Can you work these out from the drawing? Everything is in mm from the part's minimum corner. A direction names the side the tool comes from. Round coordinates to 2 decimals unless told otherwise and drop trailing zeros. Order: outer loops, then holes, each group sorted by start corner. A loop starts at its lowest first (then second) coordinate and runs counter-clockwise, first axis right, second up. Notation, with made-up numbers: M -24,65 L 5,65 A22 ccw 5,72 Z; hole C 26.25,-19 d11. An arc over 180 degrees is marked long. Write each question's results on one line, items separated by ' | '. Start each with the question number.
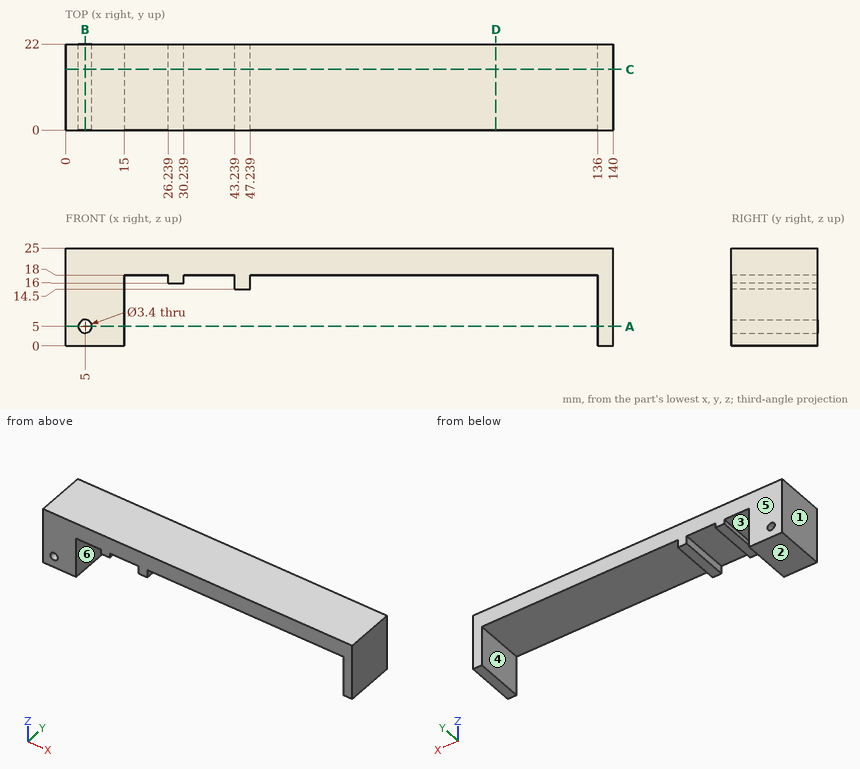
(1) I'm going to push flat-ended pins straight in: pin 1 Ø10.5 at (x, y) = (38.5, 14.5) entering from -Z; pin 2 Ø12.5 at (x, y) = (22, 14.5) entering from -Z; pin 3 Ø11 at (x, y) = (105.5, 7) entering from -Z. Where does each tip first touch, or does it pass through?
(2) I want a section at C-C on y = 15.5. Write out the boundary of the cut face in (x, z), and give its area (3 significant figures).
(3) If we mould it in two halves opening along X, with no side actions, what happens to the marked faces 1, 2, 3 and 4? For each: pulls with the +X half, pulls with the -X half, needs draft (parallel to the pull), parting line crosses it, or undercut.
(4) Please list where these lines run through material, in increasing order: line 1 (X direction, y = 16, z = 14.75); line 2 (Z direction, x = 5, y = 13.5); line 3 (X direction, y = 17.5, z = 7.25).
(5) I want a section at D-D on x = 110. Write out the boundary of the cut face in (y, z).
(6) I want a section at A-A on z = 5. Write out the boundary of the cut face in (x, y), and give its area (3 significant figures).
(7) On a 3-axis mill with a long thin cutter (end or side, diameter ignored), from which of +Z, -Z, +X, -X, +Y, -Y can I reach the whole of each face in a straight line? I mean the marked faces 5 and 6. Say none if no direction works.
(8) I want a section at B-B on x = 5. Write out the boundary of the cut face in (y, z), and give its area (3 significant figures).
Solutions:
1) pin 1: z = 14.5 | pin 2: z = 16 | pin 3: z = 18
2) outline: M 0,0 L 15,0 L 15,18 L 26.24,18 L 26.24,16 L 30.24,16 L 30.24,18 L 43.24,18 L 43.24,14.5 L 47.24,14.5 L 47.24,18 L 136,18 L 136,0 L 140,0 L 140,25 L 0,25 Z; hole C 5,5 d3.4 | area: 1,330 mm^2
3) face 1: pulls with the -X half | face 2: needs draft | face 3: undercut | face 4: undercut
4) line 1: 0 to 15, 43.24 to 47.24, 136 to 140 | line 2: 0 to 3.3, 6.7 to 25 | line 3: 0 to 15, 136 to 140
5) outline: M 0,18 L 22,18 L 22,25 L 0,25 Z
6) outline: M 0,0 L 3.3,0 L 3.3,22 L 0,22 Z; M 6.7,0 L 15,0 L 15,22 L 6.7,22 Z; M 136,0 L 140,0 L 140,22 L 136,22 Z | area: 343 mm^2
7) face 5: +Z, -Z, +X, -X, +Y | face 6: -Z, +Y, -Y
8) outline: M 0,0 L 22,0 L 22,3.3 L 0,3.3 Z; M 0,6.7 L 22,6.7 L 22,25 L 0,25 Z | area: 475 mm^2
